Check sheet for the drawn part. Datum: minimum x, y, z corner. Units: mm. Coordinates: 2 decimals unless noted, no trailing zeros. Loops run counter-clockwise (first coordinate to the right, second up) from the corner with the lowest first, then second, coordinate; pieces in that order, holes last. Notation, with made-up numbers: (-36, 39.25) - (3, 39.25) arc R12 ccw to (3, 46.25) - close; hole circle Ø1 at (-8, 62.25). An arc over 180 degrees is marked (long way). Answer as a JSON object with one key per item and string values. Group by question number.
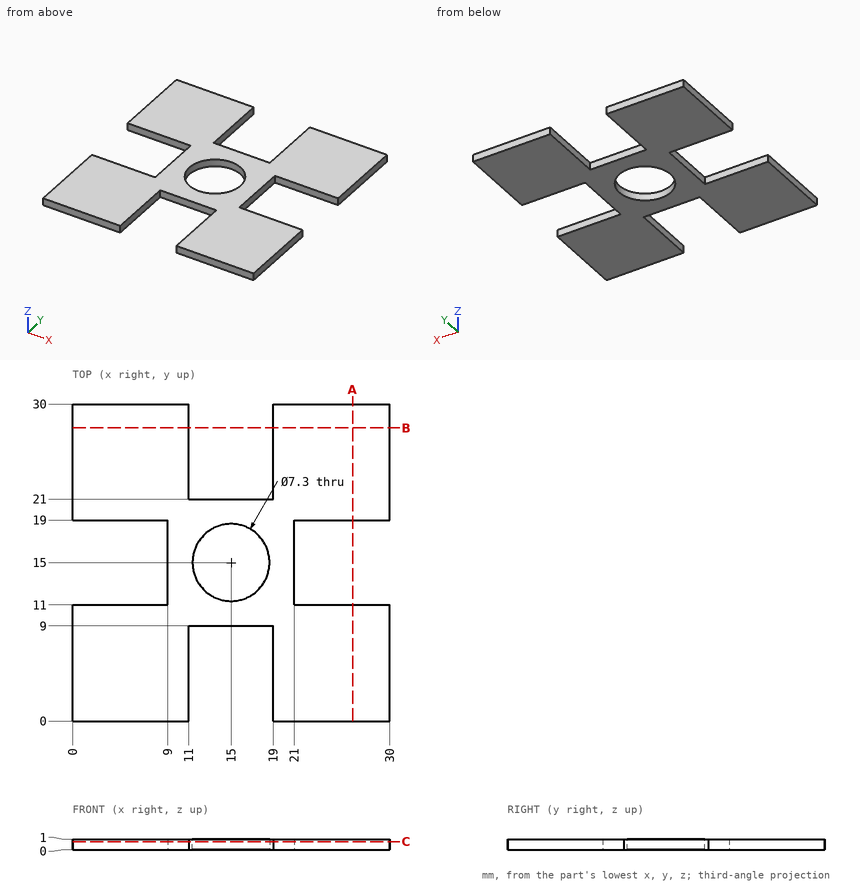
1. Sectioned sample at A-A on x = 26.5. Record the cut outline in (y, z), plus the area to 3 significant figures.
2. Gauge pin test, flat ends, axial feed: pin 1 (6.5 mm diameter, centred on x = 15, y = 15, fed in from -Z); pin 2 (0.5 mm diameter, centred on x = 14.5, z = 0.5, fed in from +Y). Record the tip position at first contact, or that the pin passes through.
3. Sectioned sample at C-C on z = 0.75. Record the cut outline in (x, y).
4. Material ranges on line 1 (Y direction, x = 15, z = 0.45); line 2 (X direction, y = 1.5, z = 0.95), recorded low to high.
Answers follow:
{
 "1": {"outline": "(0, 0) - (11, 0) - (11, 1) - (0, 1) - close; (19, 0) - (30, 0) - (30, 1) - (19, 1) - close", "area": "22.0 mm^2"},
 "2": {"pin 1": "passes through", "pin 2": "stops at y = 21"},
 "3": {"outline": "(0, 0) - (11, 0) - (11, 9) - (19, 9) - (19, 0) - (30, 0) - (30, 11) - (21, 11) - (21, 19) - (30, 19) - (30, 30) - (19, 30) - (19, 21) - (11, 21) - (11, 30) - (0, 30) - (0, 19) - (9, 19) - (9, 11) - (0, 11) - close; hole circle Ø7.3 at (15, 15)"},
 "4": {"line 1": "y = 9 to 11.35, 18.65 to 21", "line 2": "x = 0 to 11, 19 to 30"}
}
